Can you work these out from the model? Positions are in its coordinate system, mm. A direction names the side the tool comes from. Coordinates: 2 decimals unless noted, no trailing zeros. Order: outer loops, then holes, each group sorted by start corner. A loop starts at its lowest first (then second) coordinate and runs counter-clockwise, first axis right, second up. Notation, with made-up numbers: (-8.75, 1.25) -> (7.25, 1.25) arc R16 ccw to (7.25, 8.25) -> close; hole circle Ø8 at (66.5, 71.5). An arc over 180 degrees is marked (long way). Answer as a JSON object with one key per item and string values. Group by question number.
(1) I want a section at A-A, the plane z = 6.5. List the corners of the cut face in (x, y) for me.
(2) Which directions (+Z, -Z, +X, -X, +Y, -Y) give clear straight access to the entire face, cutting with the end or side of a thin tool? Please do faces 1 (the flat face through (2, 0, 0)), 2 (the flat face through (1.416, -2, -6)).
(3) I want a section at B-B, the plane x = -3.75. State how many separate pieces and enclosed holes the cut face has, plus the area to 3 significant figures.
(4) If we mould it in two halves opening along X, with no side actions, what happens to faces 3 (the flat face through (-3.119, -2.348, -0.676)), 4 (the flat face through (0, -2, 19.622)), 5 (the flat face through (9.842, -2, 0)), 6 (the flat face through (-4.54, -2.35, -2.42))? For each: pulls with the +X half, pulls with the -X half, needs draft (parallel to the pull), parting line crosses it, or undercut.
(5) I need wall thicknesses on line 1 (X direction, y = -3.6, z = 4.5); line 2 (X direction, y = -3.5, z = -15); line 3 (Z direction, x = 3, y = -0.65). Which ranges of each line are inside material? Lowest first, please.
(6) I want a section at C-C, the plane z = 13.5. List the corners of the cut face in (x, y) for me.
from build123d import *

# Parameters (mm, degrees)
F0_W     = 19.685
F0_H     = 39.243
F1_DEPTH = 4.7625


with BuildPart() as f1:
    # F0 (on Front) → F1 (new body)
    with BuildSketch(Plane.XZ):
        Rectangle(F0_W, F0_H)
        with BuildLine():
            Line((-1.416165, 10.738444), (-1.416165, 14.467826))
            Line((-1.416165, 14.467826), (1.154919, 14.467826))
            Line((1.154919, 14.467826), (1.154919, 10.738444))
            Line((1.154919, 10.738444), (8.774072, 10.738444))
            Line((8.774072, 10.738444), (8.774072, 8.923113))
            Line((8.774072, 8.923113), (1.154919, 8.923113))
            Line((1.154919, 8.923113), (1.154919, 7.524595))
            Line((1.154919, 7.524595), (5.415907, 7.524595))
            Line((5.415907, 7.524595), (5.415907, 6.059481))
            Line((5.415907, 6.059481), (1.416165, 6.059481))
            Line((1.416165, 6.059481), (1.416165, 1.835253))
            Line((1.416165, 1.835253), (4.235704, 3.396667))
            Line((4.235704, 3.396667), (4.677869, 1.835253))
            Line((4.677869, 1.835253), (1.416165, 0))
            Line((1.416165, 0), (1.416165, -11.756658))
            add(Edge.make_bspline(
                [(1.416165, -11.756658), (1.242965, -12.833442), (4.373882, -12.906026), (5.705804, -11.756658)],
                knots=[0, 0, 0, 0, 4.28964, 4.28964, 4.28964, 4.28964], degree=3))
            add(Edge.make_bspline(
                [(5.705804, -11.756658), (6.922635, -10.041888), (2.745998, -6.038307), (5.705804, -5.319911)],
                knots=[0, 0, 0, 0, 6.436747, 6.436747, 6.436747, 6.436747], degree=3))
            add(Edge.make_bspline(
                [(5.705804, -5.319911), (6.064445, -5.036285), (6.99884, -4.625151), (7.596853, -5.319911)],
                knots=[0, 0, 0, 0, 1.891049, 1.891049, 1.891049, 1.891049], degree=3))
            add(Edge.make_bspline(
                [(7.596853, -5.319911), (7.633185, -5.759441), (6.625983, -5.666271), (6.886712, -5.821177)],
                knots=[0, 0, 0, 0, 0.869234, 0.869234, 0.869234, 0.869234], degree=3))
            add(Edge.make_bspline(
                [(6.886712, -5.821177), (7.130291, -6.867712), (6.284833, -7.757668), (7.263785, -10.323707)],
                knots=[0, 0, 0, 0, 4.518291, 4.518291, 4.518291, 4.518291], degree=3))
            add(Edge.make_bspline(
                [(7.263785, -10.323707), (7.573401, -12.799004), (8.579135, -15.313338), (1.476139, -14.810471)],
                knots=[0, 0, 0, 0, 7.323106, 7.323106, 7.323106, 7.323106], degree=3))
            Line((1.476139, -14.810471), (1.491606, -15.047969))
            Line((1.491606, -15.047969), (-1.476139, -15.241242))
            Line((-1.476139, -15.241242), (-1.476139, -14.810471))
            add(Edge.make_bspline(
                [(-7.263785, -10.323707), (-7.573401, -12.799004), (-8.579135, -15.313338), (-1.476139, -14.810471)],
                knots=[0, 0, 0, 0, 7.323106, 7.323106, 7.323106, 7.323106], degree=3))
            add(Edge.make_bspline(
                [(-6.886712, -5.821177), (-7.130291, -6.867712), (-6.284833, -7.757668), (-7.263785, -10.323707)],
                knots=[0, 0, 0, 0, 4.518291, 4.518291, 4.518291, 4.518291], degree=3))
            add(Edge.make_bspline(
                [(-7.596853, -5.319911), (-7.633185, -5.759441), (-6.625983, -5.666271), (-6.886712, -5.821177)],
                knots=[0, 0, 0, 0, 0.869234, 0.869234, 0.869234, 0.869234], degree=3))
            add(Edge.make_bspline(
                [(-5.705804, -5.319911), (-6.064445, -5.036285), (-6.99884, -4.625151), (-7.596853, -5.319911)],
                knots=[0, 0, 0, 0, 1.891049, 1.891049, 1.891049, 1.891049], degree=3))
            add(Edge.make_bspline(
                [(-5.705804, -11.756658), (-6.922635, -10.041888), (-2.745998, -6.038307), (-5.705804, -5.319911)],
                knots=[0, 0, 0, 0, 6.436747, 6.436747, 6.436747, 6.436747], degree=3))
            add(Edge.make_bspline(
                [(-1.416165, -11.756658), (-1.242965, -12.833442), (-4.373882, -12.906026), (-5.705804, -11.756658)],
                knots=[0, 0, 0, 0, 4.28964, 4.28964, 4.28964, 4.28964], degree=3))
            Line((-1.416165, -11.756658), (-1.416165, -1.593658))
            Line((-1.416165, -1.593658), (-4.31391, -3.224124))
            Line((-4.31391, -3.224124), (-4.775628, -1.593658))
            Line((-4.775628, -1.593658), (-1.416165, 0.266757))
            Line((-1.416165, 0.266757), (-1.416165, 6.059481))
            Line((-1.416165, 6.059481), (-6.541871, 6.059481))
            Line((-6.541871, 6.059481), (-6.541871, 7.524595))
            Line((-6.541871, 7.524595), (-1.416165, 7.524595))
            Line((-1.416165, 7.524595), (-1.416165, 8.923113))
            Line((-1.416165, 8.923113), (-9.005928, 8.923113))
            Line((-9.005928, 8.923113), (-9.005928, 10.738444))
            Line((-9.005928, 10.738444), (-1.416165, 10.738444))
        make_face(mode=Mode.SUBTRACT)
    extrude(amount=F1_DEPTH)


solid = f1.part
Computed values:
{
 "1": {"outline": "(-9.84, -4.76) -> (-6.54, -4.76) -> (-6.54, 0) -> (-9.84, 0) -> close; (5.42, -4.76) -> (9.84, -4.76) -> (9.84, 0) -> (5.42, 0) -> close"},
 "2": {"face 1": "+Z, -Z, +X, -X, +Y", "face 2": "+Y, -Y"},
 "3": {"separate pieces": "5", "enclosed holes": "0", "area": "151 mm2"},
 "4": {"face 3": "undercut", "face 4": "needs draft", "face 5": "pulls with the +X half", "face 6": "undercut"},
 "5": {"line 1": "x = -9.84 to -1.42, 1.42 to 9.84", "line 2": "x = -9.84 to -1.48, 1.49 to 9.84", "line 3": "z = -19.62 to -14.87, -12.59 to 0.89, 2.71 to 6.06, 7.52 to 8.92, 10.74 to 19.62"},
 "6": {"outline": "(-9.84, -4.76) -> (-1.42, -4.76) -> (-1.42, 0) -> (-9.84, 0) -> close; (1.15, -4.76) -> (9.84, -4.76) -> (9.84, 0) -> (1.15, 0) -> close"}
}
